Geometry: final body of the model. Coordinates: model frame, mm. A direction names the side the tool comes from. Coordinates: 2 decimals unless noted, no trailing zeros. Loops run counter-clockwise (first coordinate to the right, second up) from the corner with the lowest first, then second, coordinate; pieces in that order, holes last. Notation, with made-up numbers: (16, 48.5) -> (55, 48.5) arc R21 ccw to (55, 74.5) -> close; hole circle Ø7 at (26.25, 84). An arc over 180 degrees is marked (long way). One line per item, written item: value. Start each with the question number.
Item 1: Ray query, probe 1 along X at (y, z) = (-3.75, 2.5); probe 2 along X at (y, z) = (3.5, 4.5); probe 3 along Z at (x, y) = (-15.5, -4.25). Return the intervals inside material, ascending. Write a range as from..to.
Item 2: Set-up query: faces 4 (the flat face through (-22, 5, 6)), 5 (the cylindrical face through (-15.5, 0.1, 6.7)), 6 (the flat face through (-19, 2, 2)), 7 (the flat face through (-17, 2, 5)). Return all of +Z, -Z, +X, -X, +Y, -Y with unobstructed straight access to the full face (end or side cutting, diameter ignored); none if empty.
Item 3: Section query B-B on y = -3.25. Return loops of the section in (x, z), then the cut area to 3 significant figures.
Item 4: Section query A-A on z = 5.25. Return loops of the section in (x, y), then the cut area to 3 significant figures.
Item 5: Mould query, pull axis X, two halves, no side actions, for faces 1 (the cylindrical face through (-13.9, 0, 1)), 2 (the flat face through (-17.8, 5, 5)), 3 (the flat face through (-24, 1, 4)). Classes: +X half, -X half, draft (parallel to the pull), parting line (faces both ways), or undercut.
Item 6: Section query C-C on z = 0.5. Return loops of the section in (x, y), then the cut area to 3 significant figures.
Item 7: Contact query for flat-ended pins moving along their axis: pin 1 Ø2.5 at (x, y) = (-24.5, -1.5) entering from -Z; pin 2 Ø1 at (y, z) = (-3.5, 4) entering from +X; pin 3 Ø1.3 at (x, y) = (-23, 3) entering from +Z. Output: stop coordinate, or through.
Item 8: Section query D-D on x = -13.5. Return loops of the section in (y, z).
from build123d import *

# Parameters (mm, degrees)
SKETCH1_R            = 1
BOSS_EXTRUDE1_DEPTH  = 6
SKETCH2_R            = 2.6
CUT_EXTRUDE1_DEPTH   = 6
SKETCH3_W            = 7.6
SKETCH3_H            = 13
BOSS_EXTRUDE2_DEPTH  = 6
BOSS_EXTRUDE5_START  = -5
SKETCH6_W            = 3
SKETCH6_H            = 2
BOSS_EXTRUDE5_DEPTH  = 13
SKETCH10_R           = 4
SKETCH10_R_2         = 2.6
BOSS_EXTRUDE6_DEPTH  = 1.5
SKETCH12_R           = 2.6
SKETCH12_R_2         = 2.4
BOSS_EXTRUDE7_DEPTH  = 2
CUT_EXTRUDE2_DEPTH   = 7
SKETCH14_W           = 3
SKETCH14_H           = 2
CUT_EXTRUDE3_DEPTH   = 7
SKETCH15_W           = 0.2
SKETCH15_H           = 13
CUT_EXTRUDE4_DEPTH   = 9.5
SKETCH16_W           = 3
SKETCH16_H           = 3
CUT_EXTRUDE5_DEPTH   = 3
BOSS_EXTRUDE8_START  = 0.2
SKETCH16_3_W         = 2.6
SKETCH16_3_H         = 2.6
BOSS_EXTRUDE8_DEPTH  = 3
BOSS_EXTRUDE9_START  = -24.2
SKETCH16_4_W         = 2.6
SKETCH16_4_H         = 2.6
BOSS_EXTRUDE9_DEPTH  = 3
SKETCH17_W           = 29.7
SKETCH17_H           = 13
CUT_EXTRUDE6_DEPTH   = 10
SKETCH18_W           = 2.6
SKETCH18_H           = 2.6
BOSS_EXTRUDE10_DEPTH = 3


with BuildPart() as part:
    # Sketch1 → Boss-Extrude1 (new body)
    with BuildSketch(Plane.XY):
        with BuildLine():
            ThreePointArc((3.75, -5), (4.47902769, -4.358991965), (5.1, -3.61282438))
            Line((5.1, -3.61282438), (5.1, 3.61282438))
            ThreePointArc((5.1, 3.61282438), (0, 6.25), (-5.1, 3.61282438))
            Line((-5.1, 3.61282438), (-5.1, -3.61282438))
            ThreePointArc((-5.1, -3.61282438), (-4.47902769, -4.358991965), (-3.75, -5))
            Line((-3.75, -5), (-14.7, -5))
            Line((-14.7, -5), (-14.7, 8))
            Line((-14.7, 8), (14.7, 8))
            Line((14.7, 8), (14.7, -5))
            Line((14.7, -5), (3.75, -5))
        make_face()
        with Locations((11.5, 0)):
            Circle(SKETCH1_R, mode=Mode.SUBTRACT)
        with Locations((-11.5, 0)):
            Circle(SKETCH1_R, mode=Mode.SUBTRACT)
    extrude(amount=BOSS_EXTRUDE1_DEPTH)

    # Sketch2 → Cut-Extrude1 (cut)
    with BuildSketch(Plane.XY):
        with Locations((-11.5, 0)):
            Circle(SKETCH2_R)
        with Locations((11.5, 0)):
            Circle(SKETCH2_R)
    extrude(amount=CUT_EXTRUDE1_DEPTH, mode=Mode.SUBTRACT)

    # Sketch3 → Boss-Extrude2 (add)
    with BuildSketch(Plane.XY):
        with Locations((-18.5, 1.5)):
            Rectangle(SKETCH3_W, SKETCH3_H)
    extrude(amount=BOSS_EXTRUDE2_DEPTH)

    # Sketch6 → Boss-Extrude5 (add)
    with BuildSketch(Plane(origin=(0, 0, 0), x_dir=(1, 0, 0), z_dir=(0, 1, 0)).offset(BOSS_EXTRUDE5_START)):
        with Locations((-23.8, -3)):
            Rectangle(SKETCH6_W, SKETCH6_H)
        with Locations((16.2, -3)):
            Rectangle(SKETCH6_W, SKETCH6_H)
    extrude(amount=BOSS_EXTRUDE5_DEPTH)

    # Sketch10 → Boss-Extrude6 (add)
    with BuildSketch(Plane.XY.offset(6)):
        with Locations((-11.5, 0)):
            Circle(SKETCH10_R)
        with Locations((-11.5, 0)):
            Circle(SKETCH10_R_2, mode=Mode.SUBTRACT)
        with BuildLine():
            Line((14.7, 2.4), (14.7, -2.4))
            ThreePointArc((14.7, -2.4), (7.5, 0), (14.7, 2.4))
        make_face()
        with Locations((11.5, 0)):
            Circle(SKETCH10_R_2, mode=Mode.SUBTRACT)
    extrude(amount=BOSS_EXTRUDE6_DEPTH)

    # Sketch12 → Boss-Extrude7 (add)
    with BuildSketch(Plane(origin=(0, 0, 0), x_dir=(-1, 0, 0), z_dir=(0, 0, -1))):
        with Locations((11.5, 0)):
            Circle(SKETCH12_R)
        with Locations((11.5, 0)):
            Circle(SKETCH12_R_2, mode=Mode.SUBTRACT)
        with Locations((-11.5, 0)):
            Circle(SKETCH12_R)
        with Locations((-11.5, 0)):
            Circle(SKETCH12_R_2, mode=Mode.SUBTRACT)
    extrude(amount=-BOSS_EXTRUDE7_DEPTH)

    # Sketch13 → Cut-Extrude2 (cut)
    with BuildSketch(Plane.XZ.offset(5)):
        Polygon((-22.3, 6), (-16.3, 6), (-16.3, 4), (-17.8, 4), (-17.8, 0), (-20.8, 0), (-20.8, 4), (-22.3, 4), align=None)
    extrude(amount=-CUT_EXTRUDE2_DEPTH, mode=Mode.SUBTRACT)

    # Sketch14 → Cut-Extrude3 (cut)
    with BuildSketch(Plane.XZ.offset(-2)):
        with Locations((-19.3, 5)):
            Rectangle(SKETCH14_W, SKETCH14_H)
    extrude(amount=-CUT_EXTRUDE3_DEPTH, mode=Mode.SUBTRACT)

    # Sketch15 → Cut-Extrude4 (cut, symmetric)
    with BuildSketch(Plane.XY):
        with Locations((-12.1, 1.5)):
            Rectangle(SKETCH15_W, SKETCH15_H)
        with Locations((12.1, 1.5)):
            Rectangle(SKETCH15_W, SKETCH15_H)
    extrude(amount=CUT_EXTRUDE4_DEPTH, both=True, mode=Mode.SUBTRACT)

    # Sketch16 → Cut-Extrude5 (cut)
    with BuildSketch(Plane.ZY.offset(12)):
        with Locations((3, 5.173669459)):
            Rectangle(SKETCH16_W, SKETCH16_H)
    cut_extrude5 = extrude(amount=-CUT_EXTRUDE5_DEPTH, mode=Mode.SUBTRACT)

    # Mirror1: Cut-Extrude5 across plane
    add(cut_extrude5.mirror(Plane(origin=(0, 0, 0), x_dir=(0, 0, 1), z_dir=(1, 0, 0))), mode=Mode.SUBTRACT)

    # Sketch16<3> → Boss-Extrude8 (add)
    with BuildSketch(Plane.ZY.offset(12).offset(BOSS_EXTRUDE8_START)):
        with Locations((3, 5.173669459)):
            Rectangle(SKETCH16_3_W, SKETCH16_3_H)
    extrude(amount=-BOSS_EXTRUDE8_DEPTH)

    # Sketch16<4> → Boss-Extrude9 (add)
    with BuildSketch(Plane.ZY.offset(12).offset(BOSS_EXTRUDE9_START)):
        with Locations((3, 5.173669459)):
            Rectangle(SKETCH16_4_W, SKETCH16_4_H)
    extrude(amount=BOSS_EXTRUDE9_DEPTH)

    # Sketch17 → Cut-Extrude6 (cut)
    with BuildSketch(Plane.XY):
        with Locations((2.85, 1.5)):
            Rectangle(SKETCH17_W, SKETCH17_H)
    extrude(amount=CUT_EXTRUDE6_DEPTH, mode=Mode.SUBTRACT)

    # Sketch18 → Boss-Extrude10 (add)
    with BuildSketch(Plane(origin=(-12.2, 0, 0), x_dir=(0, 0, -1), z_dir=(1, 0, 0))):
        with Locations((-3, 5.173669459)):
            Rectangle(SKETCH18_W, SKETCH18_H)
    extrude(amount=BOSS_EXTRUDE10_DEPTH)


solid = part.part
Reply:
1. probe 1: x = -25.3..-20.8, -17.8..-12.2
1. probe 2: x = -22.3..-20.8, -17.8..-12.2
1. probe 3: z = 0..6
2. face 4: +Z, -X, +Y, -Y
2. face 5: +Z, -X
2. face 6: +Z, -Z, -Y
2. face 7: +Z, -X, -Y
3. outline: (-25.3, 2) -> (-22.3, 2) -> (-22.3, 0) -> (-20.8, 0) -> (-20.8, 4) -> (-25.3, 4) -> close; (-17.8, 0) -> (-12.2, 0) -> (-12.2, 7.5) -> (-13.83, 7.5) -> (-13.83, 6) -> (-16.3, 6) -> (-16.3, 4) -> (-17.8, 4) -> close
3. area: 45.0 mm²
4. outline: (-22.3, 2) -> (-20.8, 2) -> (-20.8, 8) -> (-22.3, 8) -> close; (-17.8, 2) -> (-16.3, 2) -> (-16.3, -5) -> (-12.2, -5) -> (-12.2, -2.5) arc R2.6 cw to (-12.2, 2.5) -> (-12.2, 8) -> (-17.8, 8) -> close
4. area: 64.3 mm²
5. face 1: +X half
5. face 2: undercut
5. face 3: draft
6. outline: (-22.3, -5) -> (-20.8, -5) -> (-20.8, 2) -> (-17.8, 2) -> (-17.8, -5) -> (-12.2, -5) -> (-12.2, -2.3) arc R2.4 cw to (-12.2, 2.3) -> (-12.2, 8) -> (-22.3, 8) -> close
6. area: 105 mm²
7. pin 1: stops at z = 2
7. pin 2: stops at x = -12.2
7. pin 3: stops at z = 4
8. outline: (-5, 0) -> (-1.33, 0) -> (-1.33, 2) -> (-1.66, 2) -> (-1.66, 7.5) -> (-3.46, 7.5) -> (-3.46, 6) -> (-5, 6) -> close; (1.33, 0) -> (8, 0) -> (8, 6) -> (3.46, 6) -> (3.46, 7.5) -> (1.66, 7.5) -> (1.66, 2) -> (1.33, 2) -> close
